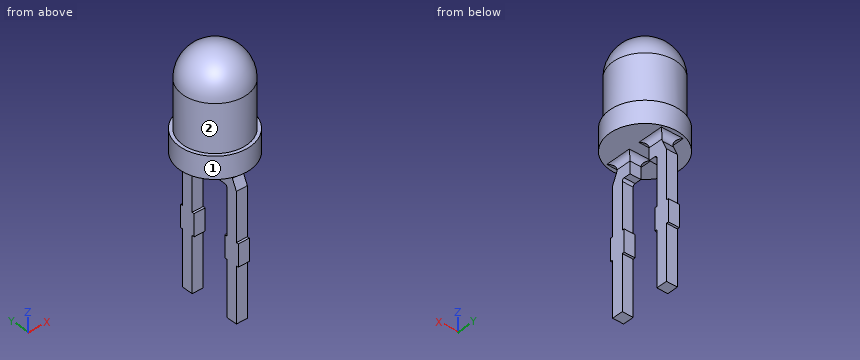
from build123d import *

# Parameters (mm, degrees)
EXTRUDE1_DEPTH          = 0.25
FILLET1_R               = 0.25
CUT_EXTRUDE1_DEPTH      = 31.234789562
CUT_EXTRUDE1_DEPTH_BACK = 31.234789562
SKETCH3_W               = 12.882415547
SKETCH3_H               = 2.8
CUT_EXTRUDE2_DEPTH      = 19.290502996
CUT_EXTRUDE2_DEPTH_BACK = 19.290502996
SKETCH4_W               = 11.746427447
SKETCH4_H               = 5.813888333


with BuildPart() as part:
    # Sketch1 → Revolve1 (revolve)
    with BuildSketch(Plane(origin=(0, 0, 0), x_dir=(0, 0, -1), z_dir=(1, 0, 0)), mode=Mode.PRIVATE) as revolve1_sk:
        with BuildLine():
            Line((0, 1.45), (2.15, 1.45))
            Line((2.15, 1.45), (2.15, 1.599999975))
            Line((2.15, 1.599999975), (3.15, 1.599999975))
            Line((3.15, 1.599999975), (3.15, 0))
            Line((3.15, 0), (-1.45, 0))
            ThreePointArc((-1.45, 0), (-1.025304833, 1.025304833), (0, 1.45))
        make_face()
    revolve(revolve1_sk.sketch.rotate(Axis((0, 0, 0), (0, 0, -1)), 90), axis=Axis((0, 0, 0), (0, 0, -1)))

    # Sketch2 → Extrude1 (add, symmetric)
    with BuildSketch(Plane(origin=(0, 0, 0), x_dir=(0, 0, -1), z_dir=(1, 0, 0))):
        with BuildLine():
            Line((3.15, 1.026953873), (3.95, 1.4))
            Line((3.95, 1.4), (6.15, 1.4))
            Line((6.15, 1.4), (6.15, 1.5))
            Line((6.15, 1.5), (7.15, 1.5))
            Line((7.15, 1.5), (7.15, 1.4))
            Line((7.15, 1.4), (30.15, 1.4))
            Line((30.15, 1.4), (30.15, 0.9))
            Line((30.15, 0.9), (7.15, 0.9))
            Line((7.15, 0.9), (7.15, 0.8))
            Line((7.15, 0.8), (6.15, 0.8))
            Line((6.15, 0.8), (6.15, 0.9))
            Line((6.15, 0.9), (4.05, 0.9))
            ThreePointArc((4.05, 0.9), (3.979289322, 0.870710678), (3.95, 0.8))
            Line((3.95, 0.8), (3.95, 0.5))
            Line((3.95, 0.5), (3.15, 0.5))
            Line((3.15, 0.5), (3.15, 1.026953873))
        make_face()
        with BuildLine():
            Line((3.95, -0.8), (3.95, -0.5))
            Line((3.95, -0.5), (3.15, -0.5))
            Line((3.15, -0.5), (3.15, -1.026953873))
            Line((3.15, -1.026953873), (3.95, -1.4))
            Line((3.95, -1.4), (6.15, -1.4))
            Line((6.15, -1.4), (6.15, -1.5))
            Line((6.15, -1.5), (7.15, -1.5))
            Line((7.15, -1.5), (7.15, -1.4))
            Line((7.15, -1.4), (30.15, -1.4))
            Line((30.15, -1.4), (30.15, -0.9))
            Line((30.15, -0.9), (7.15, -0.9))
            Line((7.15, -0.9), (7.15, -0.8))
            Line((7.15, -0.8), (6.15, -0.8))
            Line((6.15, -0.8), (6.15, -0.9))
            Line((6.15, -0.9), (4.05, -0.9))
            ThreePointArc((4.05, -0.9), (3.979289322, -0.870710678), (3.95, -0.8))
        make_face()
    extrude(amount=EXTRUDE1_DEPTH, both=True)

    # Fillet1
    fillet1_edges = [part.edges().sort_by_distance(p)[0] for p in [
        (-0.25, 0.763476937, -3.15),
        (0, 1.026953873, -3.15),
        (0, 0.5, -3.15),
        (0.25, 0.763476937, -3.15),
        (-0.25, -0.763476937, -3.15),
        (0, -0.5, -3.15),
        (0, -1.026953873, -3.15),
        (0.25, -0.763476937, -3.15),
    ]]
    fillet(fillet1_edges, radius=FILLET1_R)

    # Sketch3 → Cut-Extrude1 (cut, two sides: drawn at the far end of the back side and taken through both)
    with BuildSketch(Plane(origin=(0, 0, 0), x_dir=(0, 0, -1), z_dir=(1, 0, 0)).offset(-CUT_EXTRUDE1_DEPTH_BACK)):
        with Locations((24.591207774, 0)):
            Rectangle(SKETCH3_W, SKETCH3_H)
    extrude(amount=CUT_EXTRUDE1_DEPTH + CUT_EXTRUDE1_DEPTH_BACK, mode=Mode.SUBTRACT)

    # Sketch4 → Cut-Extrude2 (cut, two sides: drawn at the far end of the back side and taken through both)
    with BuildSketch(Plane(origin=(0, 0, 0), x_dir=(0, 0, -1), z_dir=(1, 0, 0)).offset(-CUT_EXTRUDE2_DEPTH_BACK)):
        with Locations((15.523213723, 0.186451229)):
            Rectangle(SKETCH4_W, SKETCH4_H)
    extrude(amount=CUT_EXTRUDE2_DEPTH + CUT_EXTRUDE2_DEPTH_BACK, mode=Mode.SUBTRACT)


solid = part.part
CAD build for the part. Positions are in the model's coordinates, mm. Face numbers are marked on the shaded views. A direction names the side the tool comes from. Coordinates: 2 decimals unless noted, no trailing zeros. Order: outer loops, then holes, each group sorted by start corner. A loop starts at its lowest first (then second) coordinate and runs counter-clockwise, first axis right, second up.
Item 1: Band-saw the part on D-D on z = -2.5. List the corners of the cut face in (x, y).
Check sheet entries:
outline: circle Ø3.2 at (0, 0)
Item 2: Band-saw the part on C-C on x = 1.1. List the corners of the cut face in (y, z).
Check sheet entries:
outline: (-1.16, -3.15) - (1.16, -3.15) - (1.16, -2.15) - (0.94, -2.15) - (0.94, 0) arc R0.94 ccw to (-0.94, 0) - (-0.94, -2.15) - (-1.16, -2.15) - close
Item 3: Band-saw the part on A-A on z = -7.5. List the corners of the cut face in (x, y).
Check sheet entries:
outline: (-0.25, -1.4) - (0.25, -1.4) - (0.25, -0.9) - (-0.25, -0.9) - close; (-0.25, 0.9) - (0.25, 0.9) - (0.25, 1.4) - (-0.25, 1.4) - close
Item 4: Drill centre lines: L1, parallel to Y at x = 0.1, z = -8.75; L2, parallel to X at y = -1.15, z = -6.5; L3, parallel to Z at x = -1.1, y = 0.8. Where is each one in solid material? Low to high.
Check sheet entries:
L1: y = -1.4 to -0.9, 0.9 to 1.4
L2: x = -0.25 to 0.25
L3: z = -3.15 to 0.5
Item 5: 3-axis set-ups, long thin cutter, end or side, ignore diameter. For the marked faces 1 and 2: which of +Z, -Z, +X, -X, +Y, -Y reach the whole face in a straight line?
Check sheet entries:
face 1: +Z, -Z
face 2: +Z
Item 6: Band-saw the part on B-B on y = 0. List the corners of the cut face in (x, z), plus the area to 3 significant figures.
Check sheet entries:
outline: (-1.6, -3.15) - (1.6, -3.15) - (1.6, -2.15) - (1.45, -2.15) - (1.45, 0) arc R1.45 ccw to (-1.45, 0) - (-1.45, -2.15) - (-1.6, -2.15) - close
area: 12.7 mm2
Item 7: Pin check, flat tips, straight feed: pin 1 Ø0.8 at (y, z) = (1, -5.5) entering from -X; pin 2 Ø1.5 at (x, y) = (0, 1) entering from +Z; pin 3 Ø0.6 at (x, z) = (0, -7) entering from -Y. Stop position of each tip, or through.
Check sheet entries:
pin 1: stops at x = -0.25
pin 2: stops at z = 1.43
pin 3: stops at y = -1.5
